Part model, mm, in its own coordinate system. Face numbers are marked on the shaded views. Coordinates: 2 decimals unless noted, no trailing zeros. Write each loop counter-clockwise with the first axis right and the second up, starting at its lowest first coordinate (ties: lowest second). Pieces come first, ordered by that corner, then holes. Notation, with made-up numbers: (44.25, 7) -> (102.25, 7) arc R20 cw to (102.25, 29) -> close; hole circle Ø5 at (29, 2). An arc over 180 degrees is marked (long way). One line per question, with ' | ' between items. Start each with the question number.
Item 1: Probe probe 1 along X at (y, z) = (-1.2, -2); probe 2 along Z at (x, y) = (-42.5, -2.85); probe 3 along X at (y, z) = (-1.75, 3.5). List the from-to ranges inside material, lowest first. Write a range as [from, to].
Item 2: Saw through at D-D (z = -14.25). List the corners of the cut face in (x, y), and give its area (3 significant figures).
Item 3: Saw through at B-B (z = 5.25). List the corners of the cut face in (x, y).
Item 4: Saw through at A-A (x = -14). List the corners of the cut face in (y, z), and give its area (3 significant figures).
Item 5: Pin check, flat tips, straight feed: pin 1 (0.9 mm diameter, centred on x = -0.5, y = -1, fed in from -Z); pin 2 (1.5 mm diameter, centred on y = -2, z = -10.5, fed in from +X). Stop position of each tip, or through.
Item 6: Saw through at C-C (y = -0.55). List the corners of the cut face in (x, z).
Item 7: Two-plate mould, pull along X, no slides. Class the marked faces 1, 2 and 3: pulls with the +X half, pulls with the -X half, needs draft (parallel to the pull), parting line crosses it, or undercut.
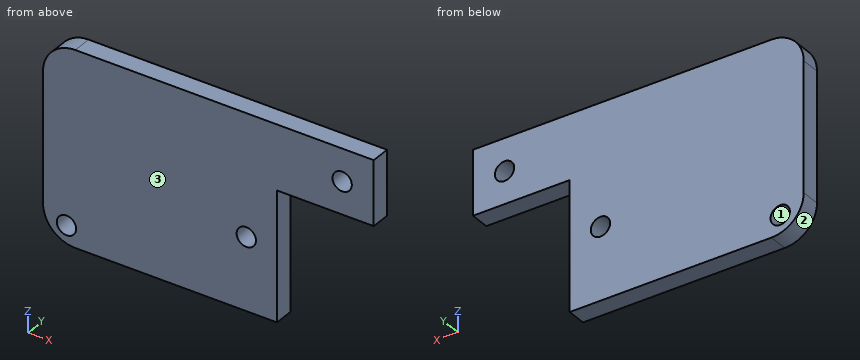
from build123d import *

# Parameters (mm, degrees)
F1_DEPTH = 3
F3_D     = 3
F4_R     = 5


with BuildPart() as f1:
    # F0 (on Front) → F1 (new body)
    with BuildSketch(Plane.XZ):
        Polygon((-45.63814, 9.742956), (-45.63814, -20.257044), (-9.356174, -20.257044), (-9.356174, -0.257044), (5.643826, -0.257044), (5.643826, 9.742956), align=None)
    extrude(amount=F1_DEPTH)

    # F3 (through all)
    with Locations(Plane.XZ.offset(3)):
        with Locations((-41.993771, -17.322723), (-14.116627, -9.033464), (0.750969, 4.742956)):
            Hole(F3_D / 2)

    # F4
    f4_edges = [f1.edges().sort_by_distance(p)[0] for p in [
        (-45.63814, -1.5, 9.742956),
        (-45.63814, -1.5, -20.257044),
    ]]
    fillet(f4_edges, radius=F4_R)


solid = f1.part
From the geometry:
1) probe 1: [-45.64, -9.36] | probe 2: [-19.9, -18.73], [-15.91, 9.38] | probe 3: [-45.64, -0.09], [1.59, 5.64]
2) outline: (-45.64, -3) -> (-9.36, -3) -> (-9.36, 0) -> (-45.64, 0) -> close | area: 109 mm2
3) outline: (-45.61, -3) -> (-0.66, -3) -> (-0.66, 0) -> (-45.61, 0) -> close; (2.16, -3) -> (5.64, -3) -> (5.64, 0) -> (2.16, 0) -> close
4) outline: (-3, -20.26) -> (0, -20.26) -> (0, -10.53) -> (-3, -10.53) -> close; (-3, -7.54) -> (0, -7.54) -> (0, 9.74) -> (-3, 9.74) -> close | area: 81.0 mm2
5) pin 1: z = -0.26 | pin 2: x = -9.36
6) outline: (-45.64, -15.26) arc R5 ccw to (-40.64, -20.26) -> (-9.36, -20.26) -> (-9.36, -0.26) -> (5.64, -0.26) -> (5.64, 9.74) -> (-40.64, 9.74) arc R5 ccw to (-45.64, 4.74) -> close; hole circle Ø3 at (-41.99, -17.32); hole circle Ø3 at (-14.12, -9.03); hole circle Ø3 at (0.75, 4.74)
7) face 1: undercut | face 2: pulls with the -X half | face 3: needs draft
